Autodesk Inventor part; units mm, degrees
ref_plane "YZ Plane" through (0, 0, 0) normal (1, 0, 0) x (0, 1, 0)
ref_plane "XZ Plane" through (0, 0, 0) normal (0, 1, 0) x (-1, 0, 0)
ref_plane "XY Plane" through (0, 0, 0) normal (0, 0, 1) x (1, 0, 0)
sketch "Sketch1" plane through (0, 0, 0) normal (0, 0, 1) x (1, 0, 0)
  circle A0 centre (0, 0) radius 8
  circle A1 centre (0, 0) radius 8
  arc A2 (-4.1289, 4.2146) -> (-5.6926, 1.5507) centre (0, 0) ccw
  line L0 (-5.6926, 1.5507) -> (-7.0866, 0.985)
  line L1 (-7.0866, 0.985) -> (-5.8997, 0.0606)
  arc A3 (-5.8997, 0.0606) -> (-5.1217, -2.9288) centre (0, 0) ccw
  line L2 (-5.1217, -2.9288) -> (-5.7075, -4.3145)
  line L3 (-5.7075, -4.3145) -> (-4.2146, -4.1289)
  arc A4 (-4.2146, -4.1289) -> (-1.5507, -5.6926) centre (0, 0) ccw
  line L4 (-1.5507, -5.6926) -> (-0.985, -7.0866)
  line L5 (-0.985, -7.0866) -> (-0.0606, -5.8997)
  arc A5 (-0.0606, -5.8997) -> (2.9288, -5.1217) centre (0, 0) ccw
  line L6 (2.9288, -5.1217) -> (4.3145, -5.7075)
  line L7 (4.3145, -5.7075) -> (4.1289, -4.2146)
  arc A6 (4.1289, -4.2146) -> (5.6926, -1.5507) centre (0, 0) ccw
  line L8 (5.6926, -1.5507) -> (7.0866, -0.985)
  line L9 (7.0866, -0.985) -> (5.8997, -0.0606)
  arc A7 (5.8997, -0.0606) -> (5.1217, 2.9288) centre (0, 0) ccw
  line L10 (5.1217, 2.9288) -> (5.7075, 4.3145)
  line L11 (5.7075, 4.3145) -> (4.2146, 4.1289)
  arc A8 (4.2146, 4.1289) -> (1.5507, 5.6926) centre (0, 0) ccw
  line L12 (1.5507, 5.6926) -> (0.985, 7.0866)
  line L13 (0.985, 7.0866) -> (0.0606, 5.8997)
  arc A9 (0.0606, 5.8997) -> (-2.9288, 5.1217) centre (0, 0) ccw
  line L14 (-2.9288, 5.1217) -> (-4.3145, 5.7075)
  line L15 (-4.3145, 5.7075) -> (-4.1289, 4.2146)
  line L16 (7.2864, -1.0128) -> (5.7765, -1.6254)
  arc A10 (4.2351, -4.2514) -> (5.7765, -1.6254) centre (0, 0) ccw
  line L17 (4.2351, -4.2514) -> (4.4361, -5.8684)
  line L18 (4.4361, -5.8684) -> (2.9353, -5.234)
  arc A11 (-0.0115, -6.0008) -> (2.9353, -5.234) centre (0, 0) ccw
  line L19 (-0.0115, -6.0008) -> (-1.0128, -7.2864)
  line L20 (-1.0128, -7.2864) -> (-1.6254, -5.7765)
  arc A12 (-4.2514, -4.2351) -> (-1.6254, -5.7765) centre (0, 0) ccw
  line L21 (-4.2514, -4.2351) -> (-5.8684, -4.4361)
  line L22 (-5.8684, -4.4361) -> (-5.234, -2.9353)
  arc A13 (-6.0008, 0.0115) -> (-5.234, -2.9353) centre (0, 0) ccw
  line L23 (-6.0008, 0.0115) -> (-7.2864, 1.0128)
  line L24 (-7.2864, 1.0128) -> (-5.7765, 1.6254)
  arc A14 (-4.2351, 4.2514) -> (-5.7765, 1.6254) centre (0, 0) ccw
  line L25 (-4.2351, 4.2514) -> (-4.4361, 5.8684)
  line L26 (-4.4361, 5.8684) -> (-2.9353, 5.234)
  arc A15 (0.0115, 6.0008) -> (-2.9353, 5.234) centre (0, 0) ccw
  line L27 (0.0115, 6.0008) -> (1.0128, 7.2864)
  line L28 (1.0128, 7.2864) -> (1.6254, 5.7765)
  arc A16 (4.2514, 4.2351) -> (1.6254, 5.7765) centre (0, 0) ccw
  line L29 (4.2514, 4.2351) -> (5.8684, 4.4361)
  line L30 (5.8684, 4.4361) -> (5.234, 2.9353)
  arc A17 (6.0008, -0.0115) -> (5.234, 2.9353) centre (0, 0) ccw
  line L31 (6.0008, -0.0115) -> (7.2864, -1.0128)
  point P0 (0, 0)
extrude "Extrusion1" add sketch "Sketch1" against normal blind 2 contours L15 L14 A9 L13 L12 A8 L11 L10 A7 L9 L8 A6 L7 L6 A5 L5 L4 A4 L3 L2 A3 L1 L0 A2
sketch "Sketch2" plane through (0, 0, 0) normal (0, 0, 1) x (1, 0, 0)
  line L0 (7.2864, -1.0128) -> (5.7765, -1.6254)
  arc A0 (4.2351, -4.2514) -> (5.7765, -1.6254) centre (0, 0) ccw
  line L1 (4.2351, -4.2514) -> (4.4361, -5.8684)
  line L2 (4.4361, -5.8684) -> (2.9353, -5.234)
  arc A1 (-0.0115, -6.0008) -> (2.9353, -5.234) centre (0, 0) ccw
  line L3 (-0.0115, -6.0008) -> (-1.0128, -7.2864)
  line L4 (-1.0128, -7.2864) -> (-1.6254, -5.7765)
  arc A2 (-4.2514, -4.2351) -> (-1.6254, -5.7765) centre (0, 0) ccw
  line L5 (-4.2514, -4.2351) -> (-5.8684, -4.4361)
  line L6 (-5.8684, -4.4361) -> (-5.234, -2.9353)
  arc A3 (-6.0008, 0.0115) -> (-5.234, -2.9353) centre (0, 0) ccw
  line L7 (-6.0008, 0.0115) -> (-7.2864, 1.0128)
  line L8 (-7.2864, 1.0128) -> (-5.7765, 1.6254)
  arc A4 (-4.2351, 4.2514) -> (-5.7765, 1.6254) centre (0, 0) ccw
  line L9 (-4.2351, 4.2514) -> (-4.4361, 5.8684)
  line L10 (-4.4361, 5.8684) -> (-2.9353, 5.234)
  arc A5 (0.0115, 6.0008) -> (-2.9353, 5.234) centre (0, 0) ccw
  line L11 (0.0115, 6.0008) -> (1.0128, 7.2864)
  line L12 (1.0128, 7.2864) -> (1.6254, 5.7765)
  arc A6 (4.2514, 4.2351) -> (1.6254, 5.7765) centre (0, 0) ccw
  line L13 (4.2514, 4.2351) -> (5.8684, 4.4361)
  line L14 (5.8684, 4.4361) -> (5.234, 2.9353)
  arc A7 (6.0008, -0.0115) -> (5.234, 2.9353) centre (0, 0) ccw
  line L15 (6.0008, -0.0115) -> (7.2864, -1.0128)
  circle A8 centre (0, 0) radius 8
  circle A9 centre (0, 0) radius 3
  line L16 (-3, 0.5) -> (3, 0.5)
  line L17 (3, 0.5) -> (3, -0.5)
  line L18 (3, -0.5) -> (-3, -0.5)
  line L19 (-3, -0.5) -> (-3, 0.5)
  line L20 (-3, 0.5) -> (3, -0.5) construction
  line L21 (3, 0.5) -> (-3, -0.5) construction
  point P0 (0, 0)
  point P1 (-3, 0)
  point P2 (-2.958, 0.5)
  point P3 (2.958, 0.5)
  point P4 (3, 0)
  point P5 (2.958, -0.5)
  point P6 (-2.958, -0.5)
  dimension "d2" = 6
  dimension "d3" = 6
  dimension "d4" = 1
extrude "Extrusion2" add sketch "Sketch2" along normal blind 1 contours L0 A0 L1 L2 A1 L3 L4 A2 L5 L6 A3 L7 L8 A4 L9 L10 A5 L11 L12 A6 L13 L14 A7 L15 | A8 | A9 L18 L16
sketch "Sketch3" plane through (0, 0, 1) normal (0, 0, 1) x (1, 0, 0)
  circle A0 centre (0, 0) radius 8
  arc A1 (-2.958, -0.5) -> (2.958, -0.5) centre (0, 0) ccw
  line L0 (-2.958, -0.5) -> (2.958, -0.5)
  line L1 (2.958, 0.5) -> (-2.958, 0.5)
  arc A2 (2.958, 0.5) -> (-2.958, 0.5) centre (0, 0) ccw
  circle A3 centre (0, 0) radius 3
  point P0 (0, 0)
  point P1 (-2.958, -0.5)
  point P2 (2.958, -0.5)
extrude "Extrusion3" add sketch "Sketch3" along normal blind 10
properties part number "handle_base_potholder"
CAD build for the part. Positions are in the model's coordinates, mm. A direction names the side the tool comes from. Round coordinates to 2 decimals unless told otherwise and drop trailing zeros. Order: outer loops, then holes, each group sorted by start corner. A loop starts at its lowest first (then second) coordinate and runs counter-clockwise, first axis right, second up. Notation, with made-up numbers: (-33.5, -16) - (-3.5, -16) arc R24 cw to (-3.5, 21) - close; hole circle Ø6 at (44.25, 84.25). An arc over 180 degrees is marked (long way). Use CSV: the item, a comma, the result in double quotes. Start each with the question number.
1) Two-plate mould, pull along X, no slides. Class faces 6 (the flat face through (6.5, -0.53, -0.99)), 7 (the flat face through (0, -0.5, 0.5)), 8 (the flat face through (3.4, 0.1, 11)): pulls with the +X half, pulls with the -X half, needs draft (parallel to the pull), parting line crosses it, or undercut.
2) Wall check: L1, parallel to Y at x = 0.25, z = 3.25; L2, parallel to Z at x = -1, y = 6.5; L3, parallel to Y at x = -2.75, z = 5. Give the ranges that are in metal, low to high. Write a range as [from, to].
3) Saw through at A-A (z = 8). List the corners of the cut face in (x, y).
4) Saw through at B-B (x = -6.5). List the corners of the cut face in (y, z), and give its area (3 significant figures).
5) Pin check, flat tips, straight feed: pin 1 Ø3 at (y, z) = (6, 7) entering from +X; pin 2 Ø0.8 at (x, y) = (0.5, -1.5) entering from +Z. Stop position of each tip, or through.
6) Tool access for faces 1 (the flat face through (6.38, -1.27, -0.99)), 2 (the flat face through (5.41, 3.61, -0.99)), 3 (the flat face through (-3.61, 5.41, -0.99)), 4 (the flat face through (1.27, 6.38, -0.99)), 5 (the cylindrical face through (-3, 0, 6)): list every direction of +Z, -Z, +X, -X, +Y, -Y with a clear straight run to the whole face (end or side of a thin tool).
Values follow:
1,face 6,"pulls with the +X half"
1,face 7,"undercut"
1,face 8,"needs draft"
2,L1,"y = [-8, -2.99], [2.99, 8]"
2,L2,"z = [0, 11]"
2,L3,"y = [-7.51, -1.2], [1.2, 7.51]"
3,outline,"circle Ø16 at (0, 0); hole (-2.96, -0.5) arc R3 ccw to (2.96, -0.5) arc R3 ccw to (2.96, 0.5) arc R3 ccw to (-2.96, 0.5) arc R3 ccw to start"
4,outline,"(-4.66, 0) - (0.53, 0) - (0.53, -2) - (1.22, -2) - (1.22, 0) - (4.66, 0) - (4.66, 11) - (-4.66, 11) - close"
4,area,"104 mm2"
5,pin 1,"stops at x = 6.61"
5,pin 2,"stops at z = 0"
6,face 1,"-Z, +X, -Y"
6,face 2,"-Z, +X"
6,face 3,"-Z, +Y"
6,face 4,"-Z, +X, +Y"
6,face 5,"+Z"
